Drawing for the job (mm, zero at the part's lowest x, y, z). A direction names the side the tool comes from. Give positions to 0.01 mm unless a question says otherwise; leave off trailing zeros. Order: outer loops, then holes, each group sorted by start corner. A loop starts at its lowest first (then second) coordinate and runs counter-clockwise, first axis right, second up. Notation, with made-up numbers: M -19,-4 L 19,-4 A19 cw 19,33 Z; hole C -6.75,6 d5. An arc over 180 degrees is marked long. Answer as a JSON object with one key per item and string values.
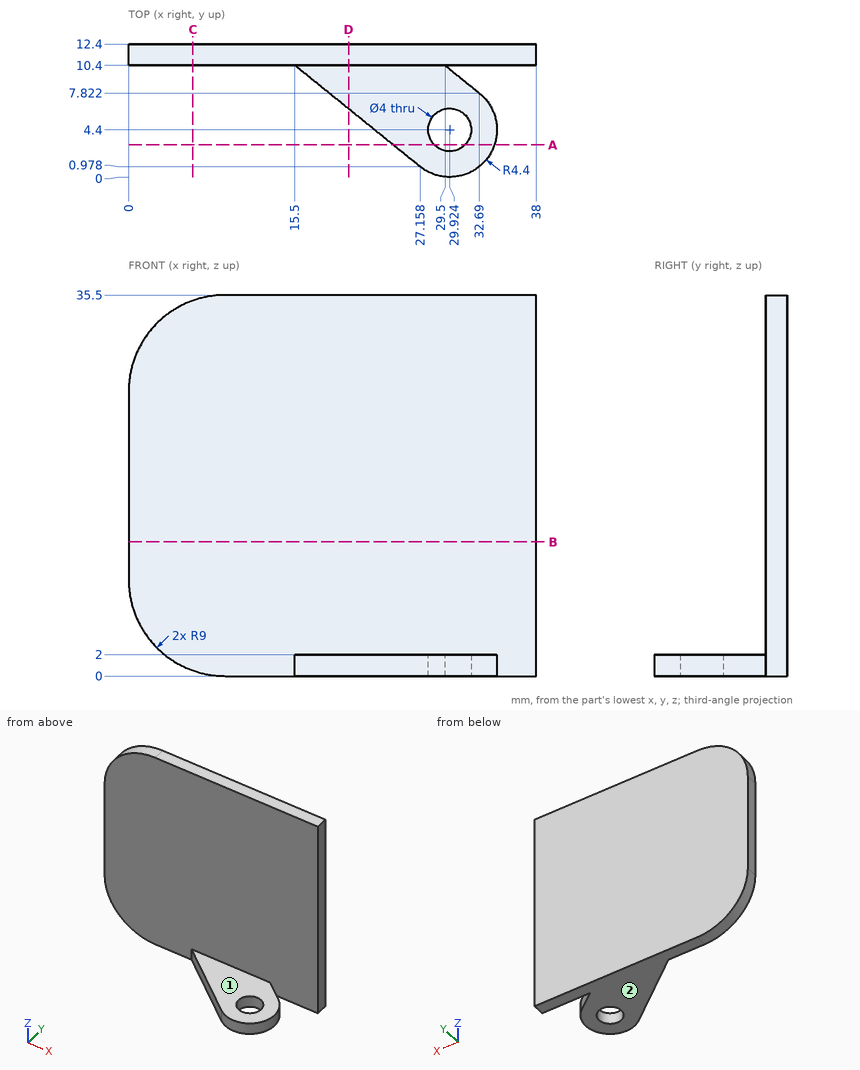
1. Cut at D-D on x = 20.5. Give the cut face in (y, z).
Worked answers:
{"outline": "M 6.36,0 L 12.4,0 L 12.4,35.5 L 10.4,35.5 L 10.4,2 L 6.36,2 Z"}
2. Pin check, flat tips, straight feed: P1, Ø12, axis at x = 23, z = 31.5, coming from the -Y side; P2, Ø2, axis at x = 30.5, y = 8, coming from the -Z side; P3, Ø2, axis at x = 15.5, y = 7.5, coming from the -Z side. Stop position of each tip, or through.
Worked answers:
{"P1": "stops at y = 10.4", "P2": "stops at z = 0", "P3": "passes through"}
3. Cut at C-C on x = 6. Give the cut face in (y, z) (1 decimal).
Worked answers:
{"outline": "M 10.4,0.5 L 12.4,0.5 L 12.4,35 L 10.4,35 Z"}
4. Cut at B-B on z = 12.5. Give the cut face in (x, y), plus the area to 3 significant figures.
Worked answers:
{"outline": "M 0,10.4 L 38,10.4 L 38,12.4 L 0,12.4 Z", "area": "76.0 mm^2"}
5. Which spindle directions (+Z, -Z, +X, -X, +Y, -Y) get a long thin tool onto all of the face, cutting with end or side? Do the marked faces 1 and 2. Say none if no direction does.
Worked answers:
{"face 1": "+Z, +X, -X, -Y", "face 2": "-Z, +X, -X, +Y, -Y"}
6. Probe line 1 along Y through (x, z) = (24, 10.5); line 2 along Z through (x, y) = (23, 9); line 3 along X through (y, z) = (10.5, 31) (1 decimal). List the from-to ranges inside material, lowest first.
Worked answers:
{"line 1": "y = 10.4 to 12.4", "line 2": "z = 0 to 2", "line 3": "x = 1.2 to 38"}
7. Cut at A-A on y = 3. Give the cut face in (x, z) (1 decimal).
Worked answers:
{"outline": "M 24.7,0 L 28.5,0 L 28.5,2 L 24.7,2 Z; M 31.4,0 L 34.1,0 L 34.1,2 L 31.4,2 Z"}
